```python
from build123d import *

# Parameters (mm, degrees)
SKETCH_W     = 15.6
SKETCH_H     = 30
PAD_DEPTH    = 13
SKETCH001_R  = 2.85
PAD001_DEPTH = 28
SKETCH002_R  = 0.75
PAD002_DEPTH = 2


with BuildPart() as part:
    # Sketch → Pad (new body)
    with BuildSketch(Plane.XY):
        with Locations((3.092153, -5.992056)):
            Rectangle(SKETCH_W, SKETCH_H)
    extrude(amount=PAD_DEPTH)

    # Sketch001 (on Face4 of Pad) → Pad001 (join)
    with BuildSketch(Plane(origin=(0, 9.007944, 0), x_dir=(-1, 0, 0), z_dir=(0, 1, 0))):
        with Locations((-2.708779, 6.233849)):
            Circle(SKETCH001_R)
    extrude(amount=PAD001_DEPTH)

    # Sketch002 (on Face3 of Pad001) → Pad002 (join)
    with BuildSketch(Plane.XZ.offset(20.992056)):
        with Locations((3.028248, 5.855581)):
            Circle(SKETCH002_R)
    extrude(amount=PAD002_DEPTH)


solid = part.part
```
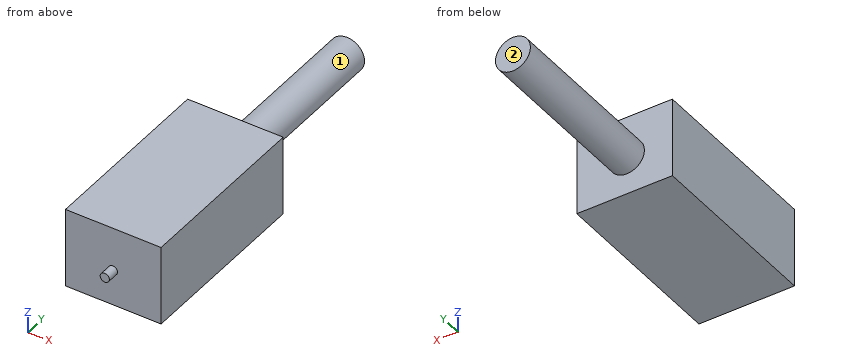
Model file for the job. Use its own axes, mm. Face numbers are marked on the shaded views. A direction names the side the tool comes from. Coordinates: 2 decimals unless noted, no trailing zeros. Order: outer loops, then holes, each group sorted by start corner. A loop starts at its lowest first (then second) coordinate and runs counter-clockwise, first axis right, second up. Notation, with made-up numbers: (53, 20) - (100, 20) arc R19 cw to (100, 25) - close; hole circle Ø10 at (-18, -27.75). An arc over 180 degrees is marked (long way). Return JSON: item names as keys, results as strings. Group by question number.
1) Saw through at A-A, the plane x = 1.75. Write the cut outline in (y, z), plus the area to 3 significant figures.
2) Saw through at D-D, the plane x = 8.5. Write the cut outline in (y, z).
3) Saw through at B-B, the plane z = 8. Write the cut outline in (x, y).
4) Tool access for the marked faces 1 and 2: list every direction of +Z, -Z, +X, -X, +Y, -Y with a clear straight run to the whole face (end or side of a thin tool).
5) Probe line 1 (Y direction, x = 10, z = 12); line 2 (Z direction, x = 2.5, y = 29); line 3 (Y direction, x = 1.5, z = 4.25). List the from-to ranges inside material, lowest first. Write a range as from..to.
6) Saw through at C-C, the plane y = 23. Write the cut outline in (x, z), plus the area to 3 significant figures.
7) Flat gauge pins, fed straight in: P1, Ø4, axis at y = 14.5, z = 7, coming from the +X side; P2, Ø5, axis at x = -0.5, z = 1.5, coming from the -Y side; P3, Ø1, axis at x = 4, y = 24, coming from the -Z side. Where does each tip first touch, or does it go through?
Values found:
{
 "1": {"outline": "(-20.99, 0) - (9.01, 0) - (9.01, 3.55) - (37.01, 3.55) - (37.01, 8.92) - (9.01, 8.92) - (9.01, 13) - (-20.99, 13) - close", "area": "540 mm²"},
 "2": {"outline": "(-20.99, 0) - (9.01, 0) - (9.01, 13) - (-20.99, 13) - close"},
 "3": {"outline": "(-4.71, -20.99) - (10.89, -20.99) - (10.89, 9.01) - (4.95, 9.01) - (4.95, 37.01) - (0.47, 37.01) - (0.47, 9.01) - (-4.71, 9.01) - close"},
 "4": {"face 1": "+Y", "face 2": "+Z, -Z, +X, -X, +Y"},
 "5": {"line 1": "y = -20.99..9.01", "line 2": "z = 3.39..9.08", "line 3": "y = -20.99..37.01"},
 "6": {"outline": "circle Ø5.7 at (2.71, 6.23)", "area": "25.5 mm²"},
 "7": {"P1": "stops at x = 5.56", "P2": "stops at y = -20.99", "P3": "stops at z = 3.5"}
}
